Work out the finished part from the listing and answer in its coordinate system (mm). A direction names the side the tool comes from. Give positions to 0.01 mm unless a question says otherwise; leave off trailing zeros. Order: outer loops, then holes, each group sorted by start corner. A loop starts at its lowest first (then second) coordinate and runs counter-clockwise, first axis right, second up. Notation, with made-up numbers: M -39.5,25.25 L -21.5,25.25 A30 ccw -21.5,50.25 Z; hole C 84,81.25 d2. An arc over 180 degrees is marked long. One line per item, written item: value.
from build123d import *

# Parameters (mm, degrees)
F1_DEPTH = 1200
F3_D     = 5
F4_R     = 2


# Not quite as in the source:
# - a feature names something its author has since deleted; it is built from what else it names


with BuildPart() as f1:
    # F0 (on Right) → F1 (new body)
    with BuildSketch(Plane.YZ):
        Polygon((-18.8378913403, 427.8021101952), (-18.8378913403, 404.8021101952), (-16.8378913403, 404.8021101952), (-16.8378913403, 429.8021101952), (-56.8378913403, 429.8021101952), (-56.8378913403, 79.8021101952), (-29.8378913403, 79.8021101952), (-29.8378913403, 53.8021101952), (-27.8378913403, 53.8021101952), (-27.8378913403, 81.8021101952), (-54.8378913403, 81.8021101952), (-54.8378913403, 427.8021101952), align=None)
    extrude(amount=F1_DEPTH)

    # F3 (through all)
    with Locations(Plane.XZ.offset(29.8378913403)):
        with Locations((433, 66.8021101952), (767, 66.8021101952), (1100, 66.8021101952), (100, 66.8021101952)):
            Hole(F3_D / 2)

    # F4
    f4_edges = [f1.edges().sort_by_distance(p)[0] for p in [
        (600, -56.837891, 429.80211),
        (600, -16.837891, 429.80211),
        (600, -56.837891, 79.80211),
        (600, -27.837891, 81.80211),
        (600, -54.837891, 81.80211),
        (600, -29.837891, 79.80211),
        (600, -18.837891, 427.80211),
        (600, -54.837891, 427.80211),
    ]]
    fillet(f4_edges, radius=F4_R)


solid = f1.part
(1) Section B-B, the plane z = 144 is taken. Give the vertices of the cut face in (x, y), then the cut area to 3 significant figures.
Findings:
outline: M 0,-56.84 L 1200,-56.84 L 1200,-54.84 L 0,-54.84 Z
area: 2,400 mm^2
(2) Determine the mould class of faces 1 (the flat face through (592, -54.838, 252)), 2 (the flat face through (592, -56.838, 257)), 3 (the flat face through (592, -37, 429.802)) for opening direction Z: pulls with the +Z half, pulls with the -Z half, needs draft (parallel to the pull), parting line crosses it, or undercut.
Findings:
face 1: undercut
face 2: needs draft
face 3: pulls with the +Z half
(3) Section A-A, the plane x = 389 is taken. Give the vertices of the cut face in (y, z), then the cut area to 3 significant figures.
Findings:
outline: M -56.84,81.8 A2 ccw -54.84,79.8 L -31.84,79.8 A2 cw -29.84,77.8 L -29.84,53.8 L -27.84,53.8 L -27.84,79.8 A2 ccw -29.84,81.8 L -52.84,81.8 A2 cw -54.84,83.8 L -54.84,425.8 A2 cw -52.84,427.8 L -20.84,427.8 A2 cw -18.84,425.8 L -18.84,404.8 L -16.84,404.8 L -16.84,427.8 A2 ccw -18.84,429.8 L -54.84,429.8 A2 ccw -56.84,427.8 Z
area: 928 mm^2
(4) Find the intervals of material crossed by probe 1 along Z at (x, y) = (767, -29.3); probe 2 along Z at (x, y) = (144, -49.5); probe 3 along Y at (x, z) = (278.5, 411), in increasing order. Write a range as from..to.
Findings:
probe 1: z = 53.8..64.3, 69.3..81.73, 427.8..429.8
probe 2: z = 79.8..81.8, 427.8..429.8
probe 3: y = -56.84..-54.84, -18.84..-16.84
(5) Given P1, Ø12, axis at x = 541.5, z = 64.5, coming from the -Y side; P2, Ø16, axis at x = 670.5, y = -37.5, coming from the -Z side; P3, Ø2, axis at x = 938.5, z = 152, coming from the +Y side; P4, Ø4, axis at x = 510.5, y = -24.5, coming from the -Z side, each flat-ended and moving along its own axis, determine where each tip first touches the part or whether it passes through.
Findings:
P1: stops at y = -29.84
P2: stops at z = 53.8
P3: stops at y = -54.84
P4: stops at z = 427.8
(6) Which of the six approach directions +Z, -Z, +X, -X, +Y, -Y give full straight-line access (tool end or side, diameter ignored) to faces 4 (the flat face through (592, -18.838, 415)), 5 (the flat face through (592, -29.838, 66)), 6 (the flat face through (592, -37, 427.802))?
Findings:
face 4: -Z, +X, -X
face 5: -Z, +X, -X, -Y
face 6: +X, -X
